Job drawing, mm, ordinate dimensions from the low corner. One solid piece. A direction names the side the tool comes from. Give positions to 0.01 mm unless a question says otherwise; leave off trailing zeros. Write each loop counter-clockwise with the first axis right and the second up, starting at its lowest first coordinate (ties: lowest second). Pieces come first, ordered by that corner, then holes. Notation, with made-up numbers: M 82.5,-25 L 127.5,-25 A16 cw 127.5,-3 Z; hole C 6,40.25 d9. An arc over 180 degrees is marked long. Answer as CSV lines item,"result". Start each with the question number.
Item 1: Band-saw the part on B-B, the plane z = 11.25. List the corners of the cut face in (x, y), then the cut area to 3 significant figures.
Item 2: Wall check: L1, parallel to X at y = 7, z = 22.25; L2, parallel to X at y = 4, z = 17. Give the ranges that are in metal, low to high. Write a range as from..to.
Item 3: Pin check, flat tip, straight feed: pin 1 (11 mm diameter, centred on x = 21.5, z = 15.5, fed in from -Y). Stop position of the tip, or through.
Item 4: 3-axis set-ups, long thin cutter, end or side, ignore diameter. For the marked faces 1 and 2: which of +Z, -Z, +X, -X, +Y, -Y reach the whole face in a straight line?
Item 5: Two-plate mould, pull along X, no slides. Class the marked faces 3, 4 and 5: +X half, -X half, draft (parallel to the pull), parting line (faces both ways), or undercut.
Item 6: Band-saw the part on A-A, the plane x = 7. List the corners of the cut face in (y, z), then the cut area to 3 significant figures.
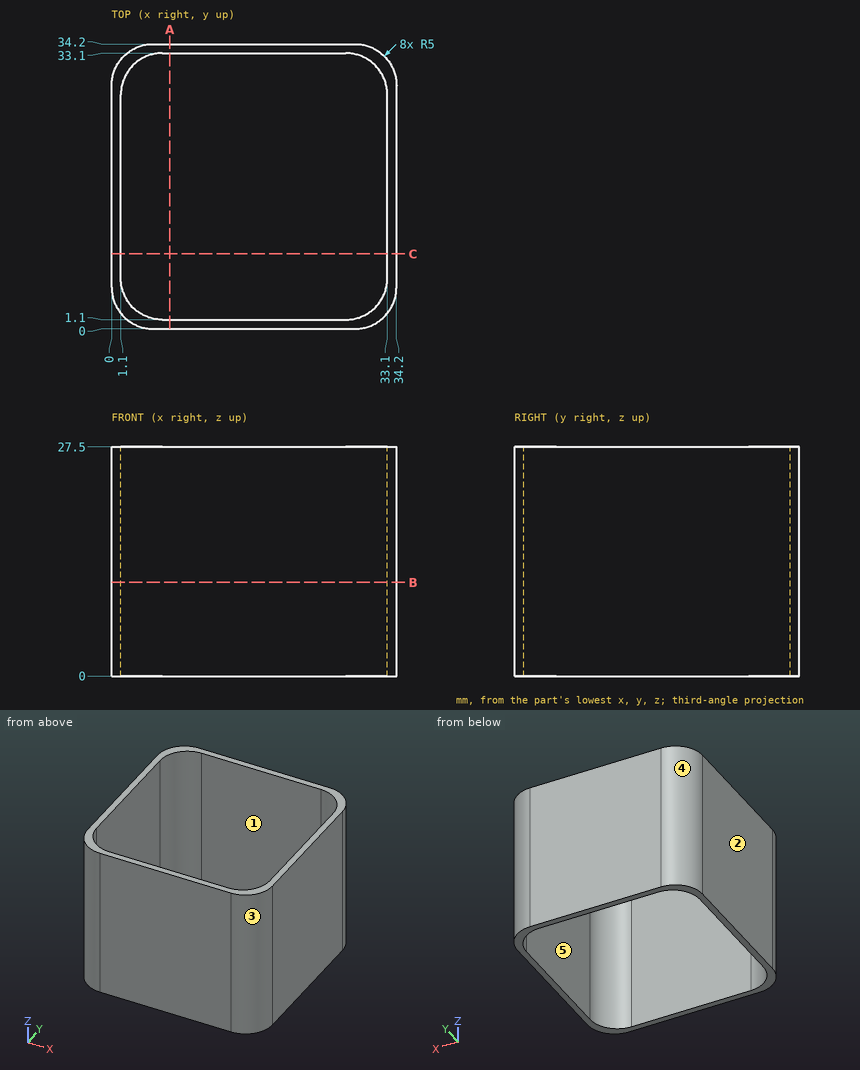
Output:
1,outline,"M 0,5 A5 ccw 5,0 L 29.2,0 A5 ccw 34.2,5 L 34.2,29.2 A5 ccw 29.2,34.2 L 5,34.2 A5 ccw 0,29.2 Z; hole M 1.1,6.1 A5 ccw 6.1,1.1 L 28.1,1.1 A5 ccw 33.1,6.1 L 33.1,28.1 A5 ccw 28.1,33.1 L 6.1,33.1 A5 ccw 1.1,28.1 Z"
1,area,"146 mm²"
2,L1,"0..1.1, 33.1..34.2"
2,L2,"0.1..1.56, 32.64..34.1"
3,pin 1,"y = 0"
4,face 1,"+Z, -Z"
4,face 2,"+Z, -Z, -X, +Y, -Y"
5,face 3,"+X half"
5,face 4,"-X half"
5,face 5,"undercut"
6,outline,"M 0,0 L 1.1,0 L 1.1,27.5 L 0,27.5 Z; M 33.1,0 L 34.2,0 L 34.2,27.5 L 33.1,27.5 Z"
6,area,"60.5 mm²"
